Input: dimensioned drawing with shaded views. Units: mm. Origin: part minimum x, y, z. Round coordinates to 2 decimals unless told otherwise and drop trailing zeros. Loops run counter-clockwise (first coordinate to the right, second up) from the corner with the lowest first, then second, coordinate; pieces in that order, holes last.
1) Section A-A, the plane y = 1.25. Return loops of the section in (x, z) (1 decimal), and give its area (3 significant figures).
2) Section C-C, the plane z = 1.1. Return loops of the section in (x, y) (1 decimal).
3) Ray query, line 1 along X through (y, z) = (1, 2.1); line 2 along X through (y, z) = (0.95, 1.05) (1 decimal); line 3 along Y through (x, z) = (41.5, 2.1). Return the intervals inside material, ascending.
4) First-contact query: pin 1 (1 mm diameter, centred on x = 51.26, y = 0.89, fed in from +Z). Flat tip, straight axial feed; report the tip coordinate or a pass-through.
5) Section B-B, the plane x = 41.5. Return loops of the section in (y, z).
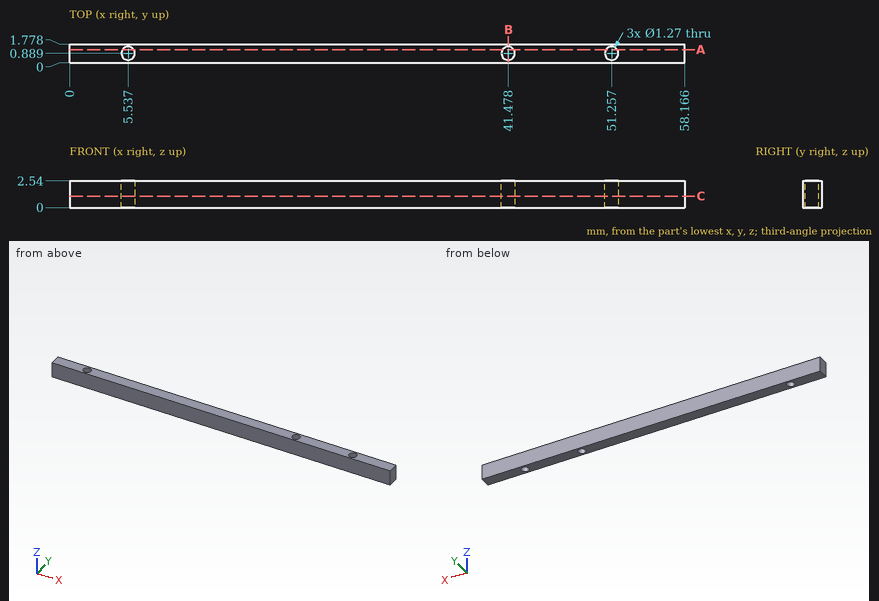
Final values:
1. outline: (0, 0) - (5, 0) - (5, 2.5) - (0, 2.5) - close; (6.1, 0) - (41, 0) - (41, 2.5) - (6.1, 2.5) - close; (42, 0) - (50.7, 0) - (50.7, 2.5) - (42, 2.5) - close; (51.8, 0) - (58.2, 0) - (58.2, 2.5) - (51.8, 2.5) - close
1. area: 140 mm2
2. outline: (0, 0) - (58.2, 0) - (58.2, 1.8) - (0, 1.8) - close; hole circle Ø1.3 at (5.5, 0.9); hole circle Ø1.3 at (41.5, 0.9); hole circle Ø1.3 at (51.3, 0.9)
3. line 1: x = 0 to 4.91, 6.16 to 40.85, 42.1 to 50.63, 51.88 to 58.17
3. line 2: x = 0 to 4.9, 6.2 to 40.8, 42.1 to 50.6, 51.9 to 58.2
3. line 3: y = 0 to 0.25, 1.52 to 1.78
4. pin 1: passes through
5. outline: (0, 0) - (0.25, 0) - (0.25, 2.54) - (0, 2.54) - close; (1.52, 0) - (1.78, 0) - (1.78, 2.54) - (1.52, 2.54) - close
